from build123d import *

# Parameters (mm, degrees)
F0_R     = 66.75
F0_R_2   = 56.75
F1_DEPTH = 45
F2_R     = 66.75
F2_R_2   = 56.75
F2_R_3   = 51.75
F3_DEPTH = 10
F6_DEPTH = 30


with BuildPart() as f1:
    # F0 (on Top) → F1 (new body)
    with BuildSketch(Plane.XY):
        Circle(F0_R)
        Circle(F0_R_2, mode=Mode.SUBTRACT)
    extrude(amount=F1_DEPTH)

    # F2 (on face) → F3 (join)
    with BuildSketch(Plane.XY.offset(45)):
        Circle(F2_R)
        Circle(F2_R_2, mode=Mode.SUBTRACT)
        Circle(F2_R_2)
        Circle(F2_R_3, mode=Mode.SUBTRACT)
    extrude(amount=-F3_DEPTH)

    # F5 (on Top) → F6 (cut)
    with BuildSketch(Plane.XY):
        with BuildLine():
            ThreePointArc((-1.8982756668, 61.7208153664), (0, 61.75), (1.8982756668, 61.7208153664))
            ThreePointArc((1.8982756668, 61.7208153664), (1.8984439159, 61.7354072521), (1.8985, 61.75))
            ThreePointArc((1.8985, 61.75), (-0.0145927479, 63.6484439159), (-1.8982756668, 61.7208153664))
        make_face()
        with BuildLine():
            ThreePointArc((-1.8982756668, 61.7208153664), (0, 59.8515), (1.8982756668, 61.7208153664))
            ThreePointArc((1.8982756668, 61.7208153664), (0, 61.75), (-1.8982756668, 61.7208153664))
        make_face()
        with BuildLine():
            ThreePointArc((61.7208153664, 1.8982756668), (61.7427034105, 0.94925), (61.75, 0))
            ThreePointArc((61.75, 0), (61.7427034105, -0.94925), (61.7208153664, -1.8982756668))
            ThreePointArc((61.7208153664, -1.8982756668), (63.0820839356, -1.3527211976), (63.6485, 0))
            ThreePointArc((63.6485, 0), (63.0820839356, 1.3527211976), (61.7208153664, 1.8982756668))
        make_face()
        with BuildLine():
            ThreePointArc((61.7208153664, -1.8982756668), (61.7427034105, -0.94925), (61.75, 0))
            ThreePointArc((61.75, 0), (61.7427034105, 0.94925), (61.7208153664, 1.8982756668))
            ThreePointArc((61.7208153664, 1.8982756668), (59.8515, 0), (61.7208153664, -1.8982756668))
        make_face()
        with BuildLine():
            ThreePointArc((1.8985, -61.75), (1.8984439159, -61.7354072521), (1.8982756668, -61.7208153664))
            ThreePointArc((1.8982756668, -61.7208153664), (0, -61.75), (-1.8982756668, -61.7208153664))
            ThreePointArc((-1.8982756668, -61.7208153664), (-0.0145927479, -63.6484439159), (1.8985, -61.75))
        make_face()
        with BuildLine():
            ThreePointArc((-1.8982756668, -61.7208153664), (0, -61.75), (1.8982756668, -61.7208153664))
            ThreePointArc((1.8982756668, -61.7208153664), (0, -59.8515), (-1.8982756668, -61.7208153664))
        make_face()
        with BuildLine():
            ThreePointArc((-59.8515, 0), (-60.3972788024, 1.3320839356), (-61.7208153664, 1.8982756668))
            ThreePointArc((-61.7208153664, 1.8982756668), (-61.75, 0), (-61.7208153664, -1.8982756668))
            ThreePointArc((-61.7208153664, -1.8982756668), (-60.3972788024, -1.3320839356), (-59.8515, 0))
        make_face()
        with BuildLine():
            ThreePointArc((-61.7208153664, -1.8982756668), (-61.75, 0), (-61.7208153664, 1.8982756668))
            ThreePointArc((-61.7208153664, 1.8982756668), (-63.6485, 0), (-61.7208153664, -1.8982756668))
        make_face()
    extrude(amount=F6_DEPTH, mode=Mode.SUBTRACT)


solid = f1.part
The listing builds one solid part. Answer for the finished solid, in the listing's coordinates (mm). A direction names the side the tool comes from. Coordinates: 2 decimals unless noted, no trailing zeros. Write each loop counter-clockwise with the first axis right and the second up, starting at its lowest first coordinate (ties: lowest second). Pieces come first, ordered by that corner, then holes. Notation, with made-up numbers: M 23,6 L 42,6 A14 cw 42,19 Z; hole C 39,76.5 d10. An arc over 180 degrees is marked long. Use one line per item in the form item = value.
Item 1: Find section C-C, the plane z = 37. Give the vertices of the cut face in (x, y).
Model answer:
outline = C 0,0 d133.5; hole C 0,0 d103.5
Item 2: Find section B-B, the plane y = -25.5. Give the vertices of the cut face in (x, z).
Model answer:
outline = M -61.69,0 L -50.7,0 L -50.7,35 L -45.03,35 L -45.03,45 L -61.69,45 Z; M 45.03,35 L 50.7,35 L 50.7,0 L 61.69,0 L 61.69,45 L 45.03,45 Z
Item 3: Find section D-D, the plane x = -50. Give the vertices of the cut face in (y, z).
Model answer:
outline = M -44.22,0 L -26.84,0 L -26.84,35 L -13.34,35 L -13.34,45 L -44.22,45 Z; M 13.34,35 L 26.84,35 L 26.84,0 L 44.22,0 L 44.22,45 L 13.34,45 Z
Item 4: Given P1, Ø5, axis at x = -51.5, z = 26, coming from the +Y side; P2, Ø1.1, axis at x = -0.5, y = 62.5, coming from the -Z side; P3, Ø4, axis at x = -28.5, z = 21.5, coming from the -Y side, each flat-ended and moving along its own axis, determine where each tip first touches the part or whether it passes through.
Model answer:
P1 = 45.33
P2 = 30
P3 = -61.26
Item 5: The mould has two halves that part along X. Classify faces 3 (the face through (-52.97, -40.62, 22.18)), 4 (the face through (-30, -49, 0)), 5 (the face through (62, 0, 30)): released by +X, released by -X, zero draft, split by the parting line, or undercut.
Model answer:
face_3 = split by the parting line
face_4 = zero draft
face_5 = undercut
Item 6: Find the intervals of material crossed by probe 1 along Y at (x, z) = (0, 40); probe 2 along Y at (x, z) = (-1, 3.5); probe 3 along X at (y, z) = (-10, 29), in increasing order.
Model answer:
probe_1 = -66.75 to -51.75, 51.75 to 66.75
probe_2 = -66.74 to -63.36, -60.14 to -56.74, 56.74 to 60.14, 63.36 to 66.74
probe_3 = -66 to -55.86, 55.86 to 66
Item 7: Find section A-A, the plane x = 0. Give the vertices of the cut face in (y, z).
Model answer:
outline = M -66.75,0 L -63.65,0 L -63.65,30 L -59.85,30 L -59.85,0 L -56.75,0 L -56.75,35 L -51.75,35 L -51.75,45 L -66.75,45 Z; M 51.75,35 L 56.75,35 L 56.75,0 L 59.85,0 L 59.85,30 L 63.65,30 L 63.65,0 L 66.75,0 L 66.75,45 L 51.75,45 Z
Item 8: For faces 1 (the face through (49.36, 15.54, 40.07)), 2 (the face through (0, 62, 30)), determine the directions among +Z, -Z, +X, -X, +Y, -Y from which every point of the face is accessible in a straight line to the end or side of a thin tool.
Model answer:
face_1 = +Z, -Z
face_2 = -Z
